CAD build for the part. Positions are in the model's coordinates, mm. Face numbers are marked on the shaded views. Round coordinates to 2 decimals unless told otherwise and drop trailing zeros. Loops run counter-clockwise (first coordinate to the right, second up) from the corner with the lowest first, then second, coordinate; pieces in that order, holes last.
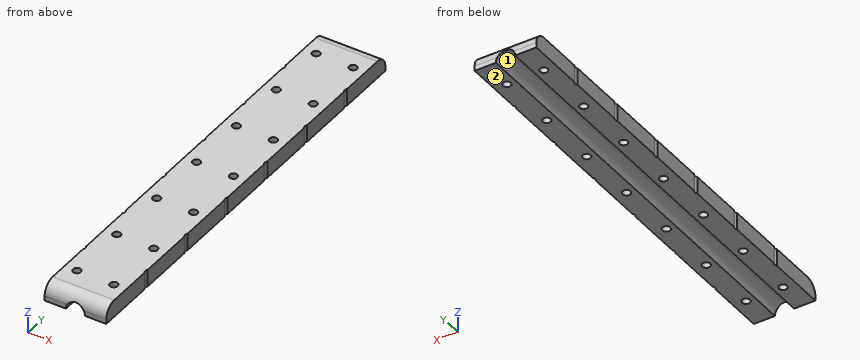
from build123d import *

# Parameters (mm, degrees)
EXTRUDE_1_DEPTH             = 87.5
SKETCH_4_R                  = 1.6
CUT_EXTRUDE_3_DEPTH         = 89.665100237
PATTERN_LINEAR_2_COUNT      = 6
PATTERN_LINEAR_2_PITCH      = 25
FILLET_1_R                  = 5
SKETCH_5_R                  = 1.6
CUT_EXTRUDE_4_DEPTH         = 89.665100357
PATTERN_LINEAR_3_COUNT      = 2
PATTERN_LINEAR_3_PITCH      = 15
PATTERN_LINEAR_3_COUNT_DIR2 = 7
PATTERN_LINEAR_3_PITCH_DIR2 = 25


with BuildPart() as part:
    # 草图2 → 凸台-拉伸1 (new, symmetric)
    with BuildSketch(Plane(origin=(0, 0, 0), x_dir=(1, 0, 0), z_dir=(0, 1, 0))):
        with BuildLine():
            Line((-3.9, 0), (-12.5, 0))
            Line((-12.5, 0), (-12.5, -7))
            Line((-12.5, -7), (12.5, -7))
            Line((12.5, -7), (12.5, 0))
            Line((12.5, 0), (3.9, 0))
            ThreePointArc((3.9, 0), (0, -3.9), (-3.9, 0))
        make_face()
    extrude(amount=EXTRUDE_1_DEPTH, both=True)

    # 草图4 → 切除-拉伸3 (cut, through all)
    with BuildSketch(Plane.XY):
        with Locations((-13.75, 62.5)):
            Circle(SKETCH_4_R)
        with Locations((13.75, 62.5)):
            Circle(SKETCH_4_R)
    cut_extrude_3 = extrude(amount=CUT_EXTRUDE_3_DEPTH, mode=Mode.SUBTRACT)

    # 阵列(线性)2: 切除-拉伸3 ×6
    with Locations(*[(0, -i * PATTERN_LINEAR_2_PITCH, 0) for i in range(1, PATTERN_LINEAR_2_COUNT)]):
        add(cut_extrude_3, mode=Mode.SUBTRACT)

    # 圆角1
    # the kernel refuses this fillet: 5 mm, written as the material it takes off along each edge
    with BuildSketch(Plane(origin=(-25, 87.5, 7), x_dir=(0, -1, 0), z_dir=(1, 0, 0))) as fillet_1_piece_1:
        with BuildLine():
            CenterArc((FILLET_1_R, FILLET_1_R), FILLET_1_R, 180, 90)
            Line((0, FILLET_1_R), (0, 0))
            Line((0, 0), (FILLET_1_R, 0))
        make_face()
    extrude(amount=50, mode=Mode.SUBTRACT)
    with BuildSketch(Plane(origin=(-25, -87.5, 7), x_dir=(0, 1, 0), z_dir=(1, 0, 0))) as fillet_1_piece_2:
        with BuildLine():
            CenterArc((FILLET_1_R, -FILLET_1_R), FILLET_1_R, 90, 90)
            Line((0, -FILLET_1_R), (0, 0))
            Line((0, 0), (FILLET_1_R, 0))
        make_face()
    extrude(amount=50, mode=Mode.SUBTRACT)

    # 草图5 → 切除-拉伸4 (cut, through all)
    with BuildSketch(Plane.XY.offset(7)):
        with Locations((-7.5, 75)):
            Circle(SKETCH_5_R)
    cut_extrude_4 = extrude(amount=-CUT_EXTRUDE_4_DEPTH, mode=Mode.SUBTRACT)

    # 阵列(线性)3: Cut-Extrude 4 2 × 7
    with Locations(*[(i * PATTERN_LINEAR_3_PITCH, -j * PATTERN_LINEAR_3_PITCH_DIR2, 0) for i in range(PATTERN_LINEAR_3_COUNT) for j in range(PATTERN_LINEAR_3_COUNT_DIR2) if (i, j) != (0, 0)]):
        add(cut_extrude_4, mode=Mode.SUBTRACT)


solid = part.part
Item 1: Cut at D-D (y = 17). List the corners of the cut face in (x, z), plus the area to 3 significant figures.
Verdict:
outline: (-12.5, 0) - (-3.9, 0) arc R3.9 cw to (3.9, 0) - (12.5, 0) - (12.5, 7) - (-12.5, 7) - close
area: 151 mm2
Item 2: Wall check: L1, parallel to X at y = -51, z = 1.5; L2, parallel to Z at x = 2, y = 3; L3, parallel to X at y = 71, z = 3.5. Give the ranges that are in metal, low to high.
Verdict:
L1: x = -12.5 to -8.75, -6.25 to -3.6, 3.6 to 6.25, 8.75 to 12.5
L2: z = 3.35 to 7
L3: x = -12.5 to -1.72, 1.72 to 12.5
Item 3: Flat gauge pin, fed straight in: P1, Ø2.5, axis at x = 7.5, y = 75, coming from the -Z side. Where does the tip first touch, or does it go through?
Verdict:
P1: passes through
Item 4: Mould opens along X. For the marked faces 1 and 2 say: released by +X, released by -X, zero draft, split by the parting line, or undercut.
Verdict:
face 1: undercut
face 2: zero draft
Item 5: Cut at B-B (x = -7.5). State how many separate pieces and enclosed holes the cut face has, plus the area to 3 significant figures.
Verdict:
separate pieces: 8
enclosed holes: 0
area: 1,060 mm2
Item 6: Cut at A-A (y = -25). List the corners of the cut face in (x, z), plus the area to 3 significant figures.
Verdict:
outline: (-12.5, 0) - (-9.1, 0) - (-9.1, 7) - (-12.5, 7) - close; (-5.9, 0) - (-3.9, 0) arc R3.9 cw to (3.9, 0) - (5.9, 0) - (5.9, 7) - (-5.9, 7) - close; (9.1, 0) - (12.5, 0) - (12.5, 7) - (9.1, 7) - close
area: 106 mm2
